Geometry check sheet. Reference: the model listing, model coordinates, mm. A direction names the side the tool comes from. Give positions to 0.01 mm unless a question says otherwise; leave off trailing zeros. Order: outer loops, then holes, each group sorted by start corner. A loop starts at its lowest first (then second) coordinate and runs counter-clockwise, first axis right, second up. Notation, with made-up numbers: M 35.5,41 L 74.5,41 A20 cw 74.5,58 Z; hole C -2,19 d1. An arc over 180 degrees is marked long. Use CSV: the item, a comma, the result in double quotes. Start each with the question number.
from build123d import *

# Parameters (mm, degrees)
SKETCH1_W                       = 60
SKETCH1_H                       = 160
BOSS_EXTRUDE1_DEPTH             = 10
BOSS_EXTRUDE2_REACH             = 32
BOSS_EXTRUDE2_DIRECTION_2_REACH = 32
CUT_EXTRUDE1_REACH              = 121.048
SKETCH3_R                       = 2.38
CHAMFER1_SIZE                   = 8
CUT_EXTRUDE2_REACH              = 12
SKETCH4_R                       = 4.5
SKETCH5_R                       = 7.5
CUT_EXTRUDE4_DEPTH              = 114.048
SKETCH6_R                       = 7.5
CUT_EXTRUDE5_DEPTH              = 5
FILLET1_R                       = 15


with BuildPart() as part:
    # Sketch1 → Boss-Extrude1 (new body)
    with BuildSketch(Plane.XY):
        Rectangle(SKETCH1_W, SKETCH1_H)
    extrude(amount=BOSS_EXTRUDE1_DEPTH)

    # Boss-Extrude2: up to this face of the body (flat: up to its plane)
    boss_extrude2_end = Plane(part.part.faces().sort_by_distance((30, 0, 5))[0])
    # Sketch2 → Boss-Extrude2 (add, up to the picked face)
    with BuildSketch(Plane(origin=(0, 0, 0), x_dir=(0, 0, -1), z_dir=(1, 0, 0)), mode=Mode.PRIVATE) as boss_extrude2_sk1:
        Polygon((0, -29.048), (0, -39.048), (85, -39.048), (85, -29.048), (0, 55.952), align=None)
    boss_extrude2_tool1 = split(extrude(boss_extrude2_sk1.sketch, amount=BOSS_EXTRUDE2_REACH, mode=Mode.PRIVATE), bisect_by=boss_extrude2_end, keep=Keep.BOTH, mode=Mode.PRIVATE)
    add(boss_extrude2_tool1.solids().sort_by_distance((0, -7.063873, -31.031746))[0])

    # Boss-Extrude2 direction 2: up to this face of the body (flat: up to its plane)
    boss_extrude2_direction_2_end = Plane(part.part.faces().sort_by_distance((-30, 0, 5))[0])
    # Sketch2 → Boss-Extrude2 direction 2 (add, up to the picked face)
    with BuildSketch(Plane(origin=(0, 0, 0), x_dir=(0, 0, -1), z_dir=(1, 0, 0)), mode=Mode.PRIVATE) as boss_extrude2_direction_2_sk1:
        Polygon((0, -29.048), (0, -39.048), (85, -39.048), (85, -29.048), (0, 55.952), align=None)
    boss_extrude2_direction_2_tool1 = split(extrude(boss_extrude2_direction_2_sk1.sketch, amount=-BOSS_EXTRUDE2_DIRECTION_2_REACH, mode=Mode.PRIVATE), bisect_by=boss_extrude2_direction_2_end, keep=Keep.BOTH, mode=Mode.PRIVATE)
    add(boss_extrude2_direction_2_tool1.solids().sort_by_distance((0, -7.063873, -31.031746))[0])

    # Sketch3 → Cut-Extrude1 (cut, up to next)
    with BuildSketch(Plane.XZ.offset(39.048), mode=Mode.PRIVATE) as cut_extrude1_sk1:
        with Locations((-10.31875, -34.75625)):
            Circle(SKETCH3_R)
    cut_extrude1_tool1 = extrude(cut_extrude1_sk1.sketch, amount=-CUT_EXTRUDE1_REACH, mode=Mode.PRIVATE) & part.part
    add(cut_extrude1_tool1.solids().sort_by_distance((-10.31875, -39.048, -34.75625))[0], mode=Mode.SUBTRACT)
    # Sketch3 → Cut-Extrude1 (cut, up to next)
    with BuildSketch(Plane.XZ.offset(39.048), mode=Mode.PRIVATE) as cut_extrude1_sk2:
        with Locations((10.31875, -34.75625)):
            Circle(SKETCH3_R)
    cut_extrude1_tool2 = extrude(cut_extrude1_sk2.sketch, amount=-CUT_EXTRUDE1_REACH, mode=Mode.PRIVATE) & part.part
    add(cut_extrude1_tool2.solids().sort_by_distance((10.31875, -39.048, -34.75625))[0], mode=Mode.SUBTRACT)
    # Sketch3 → Cut-Extrude1 (cut, up to next)
    with BuildSketch(Plane.XZ.offset(39.048), mode=Mode.PRIVATE) as cut_extrude1_sk3:
        with Locations((10.31875, -74.44375)):
            Circle(SKETCH3_R)
    cut_extrude1_tool3 = extrude(cut_extrude1_sk3.sketch, amount=-CUT_EXTRUDE1_REACH, mode=Mode.PRIVATE) & part.part
    add(cut_extrude1_tool3.solids().sort_by_distance((10.31875, -39.048, -74.44375))[0], mode=Mode.SUBTRACT)
    # Sketch3 → Cut-Extrude1 (cut, up to next)
    with BuildSketch(Plane.XZ.offset(39.048), mode=Mode.PRIVATE) as cut_extrude1_sk4:
        with Locations((-10.31875, -74.44375)):
            Circle(SKETCH3_R)
    cut_extrude1_tool4 = extrude(cut_extrude1_sk4.sketch, amount=-CUT_EXTRUDE1_REACH, mode=Mode.PRIVATE) & part.part
    add(cut_extrude1_tool4.solids().sort_by_distance((-10.31875, -39.048, -74.44375))[0], mode=Mode.SUBTRACT)

    # Chamfer1
    chamfer1_edges = [part.edges().sort_by_distance(p)[0] for p in [
        (0, -80, 0),
    ]]
    chamfer(chamfer1_edges, length=CHAMFER1_SIZE)

    # Sketch4 → Cut-Extrude2 (cut, up to next)
    with BuildSketch(Plane(origin=(0, 0, 0), x_dir=(-1, 0, 0), z_dir=(0, 0, -1)), mode=Mode.PRIVATE) as cut_extrude2_sk1:
        with Locations((-15, -60)):
            Circle(SKETCH4_R)
    cut_extrude2_tool1 = extrude(cut_extrude2_sk1.sketch, amount=-CUT_EXTRUDE2_REACH, mode=Mode.PRIVATE) & part.part
    add(cut_extrude2_tool1.solids().sort_by_distance((15, -60, 0))[0], mode=Mode.SUBTRACT)
    # Sketch4 → Cut-Extrude2 (cut, up to next)
    with BuildSketch(Plane(origin=(0, 0, 0), x_dir=(-1, 0, 0), z_dir=(0, 0, -1)), mode=Mode.PRIVATE) as cut_extrude2_sk2:
        with Locations((15, -60)):
            Circle(SKETCH4_R)
    cut_extrude2_tool2 = extrude(cut_extrude2_sk2.sketch, amount=-CUT_EXTRUDE2_REACH, mode=Mode.PRIVATE) & part.part
    add(cut_extrude2_tool2.solids().sort_by_distance((-15, -60, 0))[0], mode=Mode.SUBTRACT)
    # Sketch4 → Cut-Extrude2 (cut, up to next)
    with BuildSketch(Plane(origin=(0, 0, 0), x_dir=(-1, 0, 0), z_dir=(0, 0, -1)), mode=Mode.PRIVATE) as cut_extrude2_sk3:
        with Locations((-15, 60)):
            Circle(SKETCH4_R)
    cut_extrude2_tool3 = extrude(cut_extrude2_sk3.sketch, amount=-CUT_EXTRUDE2_REACH, mode=Mode.PRIVATE) & part.part
    add(cut_extrude2_tool3.solids().sort_by_distance((15, 60, 0))[0], mode=Mode.SUBTRACT)
    # Sketch4 → Cut-Extrude2 (cut, up to next)
    with BuildSketch(Plane(origin=(0, 0, 0), x_dir=(-1, 0, 0), z_dir=(0, 0, -1)), mode=Mode.PRIVATE) as cut_extrude2_sk4:
        with Locations((15, 60)):
            Circle(SKETCH4_R)
    cut_extrude2_tool4 = extrude(cut_extrude2_sk4.sketch, amount=-CUT_EXTRUDE2_REACH, mode=Mode.PRIVATE) & part.part
    add(cut_extrude2_tool4.solids().sort_by_distance((-15, 60, 0))[0], mode=Mode.SUBTRACT)

    # Sketch5 → Cut-Extrude4 (cut)
    with BuildSketch(Plane(origin=(0, 80, 0), x_dir=(1, 0, 0), z_dir=(0, 1, 0))):
        with Locations((-10.31875, 74.44375)):
            Circle(SKETCH5_R)
        with Locations((10.31875, 74.44375)):
            Circle(SKETCH5_R)
        with Locations((-10.31875, 34.75625)):
            Circle(SKETCH5_R)
        with Locations((10.31875, 34.75625)):
            Circle(SKETCH5_R)
    extrude(amount=-CUT_EXTRUDE4_DEPTH, mode=Mode.SUBTRACT)

    # Sketch6 → Cut-Extrude5 (cut)
    with BuildSketch(Plane(origin=(0, 0, 0), x_dir=(-1, 0, 0), z_dir=(0, 0, -1))):
        with Locations((-15, 60)):
            Circle(SKETCH6_R)
        with Locations((15, 60)):
            Circle(SKETCH6_R)
    extrude(amount=CUT_EXTRUDE5_DEPTH, mode=Mode.SUBTRACT)

    # Fillet1
    fillet1_edges = [part.edges().sort_by_distance(p)[0] for p in [
        (0, -39.048, 0),
    ]]
    fillet(fillet1_edges, radius=FILLET1_R)


solid = part.part
(1) Access from +Z, -Z, +X, -X, +Y, -Y to the whole of each face (thin tool, end or side, straight path). Record for faces 4 (the face through (-14.9, 52.5, -1.5)), 5 (the face through (9, -34.048, -37)), 6 (the face through (30, -1, -28)).
(2) Go/stop test with flat-tipped pins: P1, Ø11.5, axis at x = -15, y = -60, coming from the -Z side; P2, Ø12, axis at x = 11.5, z = -71, coming from the +Y side; P3, Ø16.5, axis at x = -7, z = -78, coming from the +Y side; P4, Ø5.5, axis at x = 15, y = 60, coming from the +Z side. Record where each tip stops, or that it passes through.
(3) Thickness scan on line 1 (X direction, y = 60, z = 7.75); line 2 (X direction, y = -39, z = -36.5); line 3 (Y direction, x = -15, z = 3.5). Record the ranges inside material, lowest first.
(4) Sectioned sample at D-D on x = -25.5. Record the cut outline in (y, z).
(5) Draft check along Z on faces 1 (the face through (-10.504, 60.198, 4.93)), 2 (the face through (0, 1, 10)), 3 (the face through (-11.945, -9.138, -27.435)). Enter one of: +Z half, -Z half, draft (parallel to the pull), parting line (faces both ways), or undercut.
(6) Sectioned sample at C-C on y = -24. Record the cut outline in (x, z).
(7) Sectioned sample at B-B on x = -15. Record the cut outline in (y, z).
(8) Sectioned sample at A-A on y = -60. Record the cut outline in (x, z), then the cut area to 3 significant figures.
Responses:
1,face 4,"-Z, +Y"
1,face 5,"+Y"
1,face 6,"+Z, -Z, +X, +Y, -Y"
2,P1,"z = 0"
2,P2,"y = -9.05"
2,P3,"y = -14.33"
2,P4,"through"
3,line 1,"-30 to -19.5, -10.5 to 10.5, 19.5 to 30"
3,line 2,"-30 to -11.94, -8.7 to 8.7, 11.94 to 30"
3,line 3,"-75.5 to -64.5, -55.5 to 55.5, 64.5 to 80"
4,outline,"M -80,8 L -72,0 L -54.05,0 A15 cw -39.05,-15 L -39.05,-85 L -29.05,-85 L 55.95,0 L 80,0 L 80,10 L -80,10 Z"
5,face 1,"draft"
5,face 2,"+Z half"
5,face 3,"undercut"
6,outline,"M -30,-79.95 L -15.41,-79.95 A7.5 cw long -5.23,-79.95 L 5.23,-79.95 A7.5 cw long 15.41,-79.95 L 30,-79.95 L 30,10 L -30,10 Z; hole C -10.32,-34.76 d15; hole C 10.32,-34.76 d15"
7,outline,"M -80,8 L -72,0 L -64.5,0 L -64.5,10 L -80,10 Z; M -55.5,0 L -54.05,0 A15 cw -39.05,-15 L -39.05,-85 L -29.05,-85 L -24.35,-80.3 L -34.05,-80.3 L -34.05,-68.58 L -12.63,-68.58 L 15.34,-40.62 L -34.05,-40.62 L -34.05,-28.9 L 27.06,-28.9 L 52.5,-3.45 L 52.5,0 L 55.5,0 L 55.5,10 L -55.5,10 Z; M 64.5,0 L 80,0 L 80,10 L 64.5,10 Z"
8,outline,"M -30,0 L -19.5,0 L -19.5,10 L -30,10 Z; M -10.5,0 L 10.5,0 L 10.5,10 L -10.5,10 Z; M 19.5,0 L 30,0 L 30,10 L 19.5,10 Z"
8,area,"420 mm2"
